from build123d import *

# Parameters (mm, degrees)
SKETCH1_W           = 104.902
SKETCH1_H           = 104.902
BOSS_EXTRUDE1_DEPTH = 2.54
SKETCH2_W           = 91.861923629
SKETCH2_H           = 104.902
SKETCH2_W_2         = 7.806745179
BOSS_EXTRUDE2_DEPTH = 14.732
SKETCH3_R           = 1.778
CUT_EXTRUDE1_DEPTH  = 18.272
SKETCH4_W           = 68.459098584
SKETCH4_H           = 14.819221787
SKETCH4_H_2         = 13.598803865
SKETCH4_W_2         = 14.616932407
BOSS_EXTRUDE3_DEPTH = 11.43


with BuildPart() as part:
    # Sketch1 → Boss-Extrude1 (new body)
    with BuildSketch(Plane(origin=(0, 0, 0), x_dir=(1, 0, 0), z_dir=(0, 1, 0))):
        with Locations((52.451, 52.451)):
            Rectangle(SKETCH1_W, SKETCH1_H)
    extrude(amount=BOSS_EXTRUDE1_DEPTH)

    # Sketch2 → Boss-Extrude2 (add)
    with BuildSketch(Plane(origin=(0, 2.54, 0), x_dir=(1, 0, 0), z_dir=(0, 1, 0))):
        with Locations((58.971038185, 52.451)):
            Rectangle(SKETCH2_W, SKETCH2_H)
        with Locations((3.90337259, 52.451)):
            Rectangle(SKETCH2_W_2, SKETCH2_H)
    extrude(amount=BOSS_EXTRUDE2_DEPTH)

    # Sketch3 → Cut-Extrude1 (cut, through all)
    with BuildSketch(Plane(origin=(0, 17.272, 0), x_dir=(1, 0, 0), z_dir=(0, 1, 0))):
        with Locations((98.298, 6.604)):
            Circle(SKETCH3_R)
        with Locations((98.298, 98.298)):
            Circle(SKETCH3_R)
        with Locations((19.304, 6.604)):
            Circle(SKETCH3_R)
        with Locations((19.304, 98.298)):
            Circle(SKETCH3_R)
    extrude(amount=-CUT_EXTRUDE1_DEPTH, mode=Mode.SUBTRACT)

    # Sketch4 → Boss-Extrude3 (add)
    with BuildSketch(Plane.XZ):
        with Locations((58.99120595, -97.492389107)):
            Rectangle(SKETCH4_W, SKETCH4_H)
        with Locations((58.99120595, -6.799401933)):
            Rectangle(SKETCH4_W, SKETCH4_H_2)
        with Locations((7.308466204, -6.799401933)):
            Rectangle(SKETCH4_W_2, SKETCH4_H_2)
    extrude(amount=BOSS_EXTRUDE3_DEPTH)


solid = part.part
Read the model definition and answer for the solid it produces. Units are mm, in the model's axes. A direction names the side the tool comes from. Round coordinates to 2 decimals unless told otherwise and drop trailing zeros. Order: outer loops, then holes, each group sorted by start corner. A loop starts at its lowest first (then second) coordinate and runs counter-clockwise, first axis right, second up.
1) Flat-ended cylindrical pins translate along their axes: pin 1 (12.5 mm diameter, centred on x = 8, y = -3, fed in from -Z); pin 2 (9 mm diameter, centred on y = -6.5, z = -100.5, fed in from +X); pin 3 (1 mm diameter, centred on x = 37.5, z = -30.5, fed in from -Y); pin 4 (2.5 mm diameter, centred on x = 10, z = -73, fed in from +Y). Find the tip coordinate at first contact, or state that the pin passes through.
2) The part is cut by section C-C on x = 72. Write down the section's boundary in (y, z).
3) The part is cut by section A-A on y = -9.5. Write down the section's boundary in (x, z), plus the area to 3 significant figures.
4) The part is cut by section D-D on z = -42. Write down the section's boundary in (x, y), plus the area to 3 significant figures.
5) The part is cut by section B-B on y = 8.5. Write down the section's boundary in (x, z).
6) For faces 1 (the face through (10, 2.54, -53)), 2 (the face through (93.221, -6, -98)), 3 (the face through (59, -6, -13.599)), 4 (the face through (24.762, -6, -7)), determine the directions among +Z, -Z, +X, -X, +Y, -Y from which every point of the face is accessible in a straight line to the end or side of a thin tool.
7) Straight lines are drawn through the part: L1, parallel to Z at x = 57.5, y = -6.5; L2, parallel to X at y = 15, z = -72.5; L3, parallel to Y at x = 57.5, z = -20. For each, find the intervals that lie inside material, in ascending order.
Resolved:
1. pin 1: stops at z = -104.9
1. pin 2: stops at x = 93.22
1. pin 3: stops at y = 0
1. pin 4: stops at y = 2.54
2. outline: (-11.43, -104.9) - (17.27, -104.9) - (17.27, 0) - (-11.43, 0) - (-11.43, -13.6) - (0, -13.6) - (0, -90.08) - (-11.43, -90.08) - close
3. outline: (0, -13.6) - (14.62, -13.6) - (14.62, 0) - (0, 0) - close; (24.76, -104.9) - (93.22, -104.9) - (93.22, -90.08) - (24.76, -90.08) - close; (24.76, -13.6) - (93.22, -13.6) - (93.22, 0) - (24.76, 0) - close
3. area: 2,140 mm2
4. outline: (0, 0) - (104.9, 0) - (104.9, 17.27) - (13.04, 17.27) - (13.04, 2.54) - (7.81, 2.54) - (7.81, 17.27) - (0, 17.27) - close
4. area: 1,730 mm2
5. outline: (0, -104.9) - (7.81, -104.9) - (7.81, 0) - (0, 0) - close; (13.04, -104.9) - (104.9, -104.9) - (104.9, 0) - (13.04, 0) - close; hole circle Ø3.56 at (19.3, -98.3); hole circle Ø3.56 at (19.3, -6.6); hole circle Ø3.56 at (98.3, -98.3); hole circle Ø3.56 at (98.3, -6.6)
6. face 1: +Z, -Z, +Y
6. face 2: +Z, -Z, +X, -Y
6. face 3: +X, -X, -Y
6. face 4: +Z, -Z, -Y
7. L1: z = -104.9 to -90.08, -13.6 to 0
7. L2: x = 0 to 7.81, 13.04 to 104.9
7. L3: y = 0 to 17.27
